Verification items for the finished model (mm, model axes). A direction names the side the tool comes from. Coordinates: 2 decimals unless noted, no trailing zeros. Order: outer loops, then holes, each group sorted by start corner. A loop starts at its lowest first (then second) coordinate and runs counter-clockwise, first axis right, second up. Notation, with made-up numbers: (68, -31.75) -> (122, -31.75) arc R16 cw to (122, -10.75) -> close; hole circle Ø7 at (15.25, 69). An arc over 180 degrees is marked (long way). Write each question's results on one line, items separated by ' | '. Start each with the question number.
(1) Cross-section at C-C on x = 38.5. Enter the section's corners in (y, z).
(2) Cross-section at D-D on y = 7.5. Enter the section's corners in (x, z).
(3) Go/stop test with flat-tipped pins: pin 1 (2.5 mm diameter, centred on x = -21.5, y = 2, fed in from +Z); pin 2 (1 mm diameter, centred on x = 8.5, z = 3.5, fed in from +Y); pin 3 (10 mm diameter, centred on x = 45, y = -13, fed in from -Z). Record where each tip stops, or that it passes through.
(4) Set-up check for faces 1 (the flat face through (74.6, -14.2, 4)), 2 (the flat face through (72, -14, 2)): record each of +Z, -Z, +X, -X, +Y, -Y from which the full face is reachable in a straight line by a thin tool's end or side.
(5) Thickness scan on probe 1 along X at (y, z) = (-13, 3.25); probe 2 along X at (y, z) = (-1, 3.6); probe 3 along Z at (x, y) = (-63.5, -0.5). Record the ranges inside material, lowest first. Write a range as [from, to].
(6) Cross-section at B-B on y = 15. Enter the section's corners in (x, z), and give its area (3 significant figures).
(7) Cross-section at A-A on z = 3.1. Give the number of separate pieces and of enclosed holes in the cut face, and give its area (4 significant figures).
(8) Draft check along Y on faces 3 (the flat face through (-69, -14, 4)), 4 (the flat face through (72, 14, 2)), 5 (the flat face through (-1, 17.5, 1)). Enter one of: +Y half, -Y half, draft (parallel to the pull), parting line (faces both ways), or undercut.
```python
from build123d import *

# Parameters (mm, degrees)
SKICA1_W                = 150
SKICA1_H                = 35
P_IDAT_VYSUNUT_M2_DEPTH = 2
SKICA2_W                = 6.5
SKICA2_H                = 11.5
SKICA2_W_2              = 5
SKICA2_H_2              = 10
P_IDAT_VYSUNUT_M3_DEPTH = 2
SKICA3_W                = 6.5
SKICA3_H                = 6.5
SKICA3_W_2              = 5
SKICA3_H_2              = 5
P_IDAT_VYSUNUT_M4_DEPTH = 2


with BuildPart() as part:
    # Skica1 → Přidat vysunutím2 (new body)
    with BuildSketch(Plane.XY):
        Rectangle(SKICA1_W, SKICA1_H)
    extrude(amount=P_IDAT_VYSUNUT_M2_DEPTH)

    # Skica2 → Přidat vysunutím3 (add)
    with BuildSketch(Plane.XY.offset(2)):
        with Locations((-22.5, 0)):
            Rectangle(SKICA2_W, SKICA2_H)
        with Locations((-22.5, 0)):
            Rectangle(SKICA2_W_2, SKICA2_H_2, mode=Mode.SUBTRACT)
        with Locations((9.5, 0)):
            Rectangle(SKICA2_W, SKICA2_H)
        with Locations((9.5, 0)):
            Rectangle(SKICA2_W_2, SKICA2_H_2, mode=Mode.SUBTRACT)
    extrude(amount=P_IDAT_VYSUNUT_M3_DEPTH)

    # Skica3 → Přidat vysunutím4 (add)
    with BuildSketch(Plane.XY.offset(2)):
        with Locations((-71.75, 14.25)):
            Rectangle(SKICA3_W, SKICA3_H)
        with Locations((-71.75, 14.25)):
            Rectangle(SKICA3_W_2, SKICA3_H_2, mode=Mode.SUBTRACT)
        with Locations((71.75, 14.25)):
            Rectangle(SKICA3_W, SKICA3_H)
        with Locations((71.75, 14.25)):
            Rectangle(SKICA3_W_2, SKICA3_H_2, mode=Mode.SUBTRACT)
        with Locations((-71.75, -14.25)):
            Rectangle(SKICA3_W, SKICA3_H)
        with Locations((-71.75, -14.25)):
            Rectangle(SKICA3_W_2, SKICA3_H_2, mode=Mode.SUBTRACT)
        with Locations((71.75, -14.25)):
            Rectangle(SKICA3_W, SKICA3_H)
        with Locations((71.75, -14.25)):
            Rectangle(SKICA3_W_2, SKICA3_H_2, mode=Mode.SUBTRACT)
    extrude(amount=P_IDAT_VYSUNUT_M4_DEPTH)


solid = part.part
```
Results are:
1) outline: (-17.5, 0) -> (17.5, 0) -> (17.5, 2) -> (-17.5, 2) -> close
2) outline: (-75, 0) -> (75, 0) -> (75, 2) -> (-75, 2) -> close
3) pin 1: stops at z = 2 | pin 2: stops at y = 5.75 | pin 3: stops at z = 0
4) face 1: +Z, +X, -X, +Y, -Y | face 2: +Z
5) probe 1: x = [-75, -74.25], [-69.25, -68.5], [68.5, 69.25], [74.25, 75] | probe 2: x = [-25.75, -25], [-20, -19.25], [6.25, 7], [12, 12.75] | probe 3: z = [0, 2]
6) outline: (-75, 0) -> (75, 0) -> (75, 4) -> (74.25, 4) -> (74.25, 2) -> (69.25, 2) -> (69.25, 4) -> (68.5, 4) -> (68.5, 2) -> (-68.5, 2) -> (-68.5, 4) -> (-69.25, 4) -> (-69.25, 2) -> (-74.25, 2) -> (-74.25, 4) -> (-75, 4) -> close | area: 306 mm2
7) separate pieces: 6 | enclosed holes: 6 | area: 118.5 mm2
8) face 3: draft | face 4: undercut | face 5: +Y half
